Read the model definition and answer for the solid it produces. Units are mm, in the model's axes. Face numbers are marked on the shaded views. A direction names the side the tool comes from. Coordinates: 2 decimals unless noted, no trailing zeros. Write each loop counter-clockwise with the first axis right and the second up, starting at its lowest first coordinate (ties: lowest second). Pieces come first, ordered by that corner, then holes. Notation, with made-up numbers: (62, 53.25) -> (110, 53.25) arc R22 ccw to (110, 92.25) -> close; hole circle Ø4 at (-24.5, 15.25). An arc over 180 degrees is marked (long way). Use CSV: the item, a comma, the result in double quotes. Start each with the question number.
from build123d import *

# Parameters (mm, degrees)
F0_R     = 26
F0_R_2   = 16
F1_DEPTH = 20
F2_DEPTH = 12
F3_W     = 52
F3_H     = 17
F4_DEPTH = 2


with BuildPart() as f1:
    # F0 (on Top) → F1 (new body)
    with BuildSketch(Plane.XY):
        Circle(F0_R)
        Circle(F0_R_2, mode=Mode.SUBTRACT)
        Circle(F0_R_2)
    extrude(amount=-F1_DEPTH)

    # F0 (on Top) → F2 (cut)
    with BuildSketch(Plane.XY):
        Circle(F0_R_2)
    extrude(amount=-F2_DEPTH, mode=Mode.SUBTRACT)

    # F3 (on Top) → F4 (cut)
    with BuildSketch(Plane.XY):
        Rectangle(F3_W, F3_H)
    extrude(amount=-F4_DEPTH, mode=Mode.SUBTRACT)


solid = f1.part
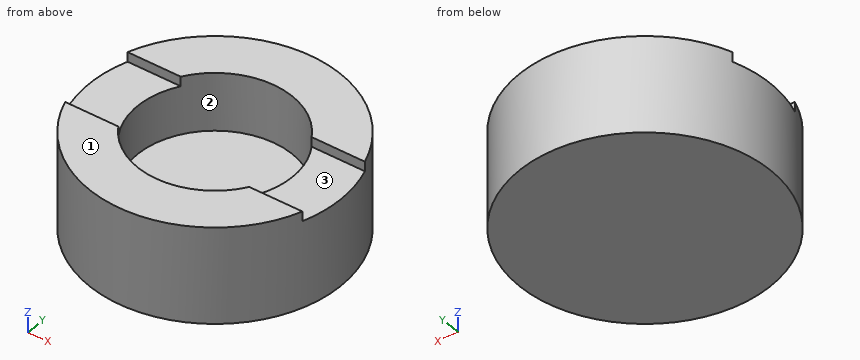
1) Each of these flat-tipped pins is pushed along its axis until it touches: pin 1 (2 mm diameter, centred on x = 18, z = -0.5, fed in from +Y); pin 2 (8 mm diameter, centred on x = 20.5, z = -8.5, fed in from -Y); pin 3 (3.5 mm diameter, centred on x = 22.5, y = 2, fed in from +Z). Where does it stop, or does it pass through?
2) Section C-C, the plane z = -3 is taken. Give the vertices of the cut face in (x, y).
3) Section B-B, the plane x = -10 is taken. Give the vertices of the cut face in (y, z), plus the area to 3 significant figures.
4) Section D-D, the plane z = -17.25 is taken. Give the vertices of the cut face in (x, y).
5) Section A-A, the plane y = 0 is taken. Give the vertices of the cut face in (x, z), plus the area to 3 significant figures.
6) Find the intervals of material crossed by line 1 along Y through (x, z) = (0, -3); line 2 along X through (y, z) = (-8, -8); line 3 along Y through (x, z) = (10.5, -1), in increasing order.
7) Which of the six approach directions +Z, -Z, +X, -X, +Y, -Y give full straight-line access (tool end or side, diameter ignored) to the marked faces 1, 2 and 3?
The answers:
1,pin 1,"stops at y = 19.67"
1,pin 2,"stops at y = -20.09"
1,pin 3,"stops at z = -2"
2,outline,"circle Ø52 at (0, 0); hole circle Ø32 at (0, 0)"
3,outline,"(-24, -20) -> (24, -20) -> (24, 0) -> (12.49, 0) -> (12.49, -12) -> (-12.49, -12) -> (-12.49, 0) -> (-24, 0) -> close"
3,area,"660 mm^2"
4,outline,"circle Ø52 at (0, 0)"
5,outline,"(-26, -20) -> (26, -20) -> (26, -2) -> (16, -2) -> (16, -12) -> (-16, -12) -> (-16, -2) -> (-26, -2) -> close"
5,area,"616 mm^2"
6,line 1,"y = -26 to -16, 16 to 26"
6,line 2,"x = -24.74 to -13.86, 13.86 to 24.74"
6,line 3,"y = -23.79 to -12.07, 12.07 to 23.79"
7,face 1,"+Z, +X, -X, +Y, -Y"
7,face 2,"+Z"
7,face 3,"+Z, +X, -X"
